Autodesk Fusion 360 part; units mm, degrees
sketch "Sketch1" plane through (0, 0, 0) normal (1, 0, 0) x (0, 1, 0)
  line L0 (0, 0) -> (35, 0)
  line L1 (35, 0) -> (35, -23)
  line L2 (35, -23) -> (40, -23)
  line L3 (0, 0) -> (0, 10)
  line L4 (15, 30.2) -> (15, 10)
  line L5 (15, 10) -> (40, 10)
  line L6 (40, 10) -> (40, -23)
  line L7 (0, 10) -> (0, 30)
  line L8 (0, 30) -> (0, 40)
  line L9 (0, 40) -> (15, 40)
  line L10 (15, 40) -> (15, 30.2)
  line L11 (15, 10) -> (15, 28.5) construction
  line L12 (15, 28.5) -> (35, 10)
  dimension "d1" = 35
  dimension "d2" = 23
  dimension "d3" = 5
  dimension "d4" = 10
  dimension "d8" = 20.2
  dimension "d9" = 20
  dimension "d10" = 10
  dimension "d19" = 18.5
extrude "Extrude1" add sketch "Sketch1" along normal blind 40 contours L0 L1 L2 L3 L4 L5 L6 L7 L8 L9 L10
sketch "Sketch2" plane through (0, 0, 0) normal (0, -1, 0) x (1, 0, 0)
  line L0 (0, 40) -> (0, 0)
  line L1 (0, 0) -> (40, 0)
  line L2 (40, 0) -> (40, 40)
  line L3 (40, 40) -> (0, 40)
  line L4 (29.815, 20) -> (24.9075, 28.5)
  line L5 (24.9075, 28.5) -> (15.0925, 28.5)
  line L6 (15.0925, 28.5) -> (10.185, 20)
  line L7 (10.185, 20) -> (15.0925, 11.5)
  line L8 (15.0925, 11.5) -> (24.9075, 11.5)
  line L9 (24.9075, 11.5) -> (29.815, 20)
  line L10 (0, 20) -> (40, 20) construction
  line L11 (20, 40) -> (20, 0) construction
  circle A0 centre (20, 20) radius 5.1
  line L12 (0, 0) -> (0, -11.5) construction
  line L13 (0, -11.5) -> (10, -11.5) construction
  line L14 (10, -11.5) -> (20, -11.5) construction
  circle A1 centre (20, -11.5) radius 2.1
  point P0 (20, 20)
  point P1 (20, 20)
  dimension "d13" = 8.5
  dimension "d14" = 10.2
  dimension "d25" = 11.5
  dimension "d26" = 10
  dimension "d27" = 4.2
extrude "Extrude2" cut sketch "Sketch2" against normal through all contours A0 | A1
extrude "Extrude3" cut sketch "Sketch2" along normal blind 7.5 from surface at -15 contours L4 L5 L6 L7 L8 L9
extrude "Extrude4" add sketch "Sketch1" along normal blind 4 contours L4 L5 L12
extrude "Extrude5" add sketch "Sketch1" against normal blind 4 from surface at 40 contours L4 L5 L12
sketch "Sketch3" plane through (0, 0, 10) normal (0, 0, 1) x (-1, 0, 0)
  line L0 (-36, -35) -> (-40, -35)
  line L1 (-40, -35) -> (-40, -40)
  line L2 (-40, -40) -> (0, -40)
  line L3 (0, -40) -> (0, -35)
  line L4 (0, -35) -> (-4, -35)
  line L5 (-4, -35) -> (-4, -15)
  line L6 (-4, -15) -> (-36, -15)
  line L7 (-36, -15) -> (-36, -35)
  line L8 (0, -40) -> (-10, -40) construction
  line L9 (-10, -40) -> (-10, -27.5) construction
  circle A0 centre (-10, -27.5) radius 1.6
  line L10 (-10, -27.5) -> (-30, -27.5) construction
  circle A1 centre (-30, -27.5) radius 1.6
  dimension "d28" = 10
  dimension "d29" = 12.5
  dimension "d30" = 3.2
  dimension "d31" = 20
  dimension "d32" = 3.2
extrude "Extrude6" cut sketch "Sketch3" along normal through all contours A0 | A1
equation "d8 = 30.200 mm - 10 mm"
equation "d13 = ( 17 / 2 ) * 1 mm"
equation "d19 = 28.50 mm - 10 mm"
equation "d25 = ( 23 / 2 ) * 1 mm"
equation "d29 = ( 25 / 2 ) * 1 mm"
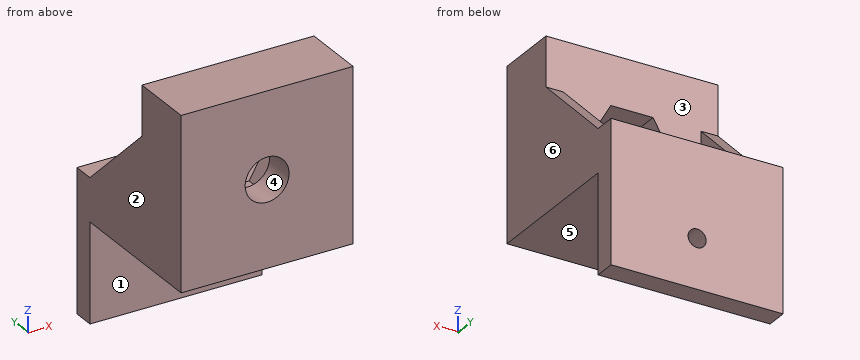
For this review, take the finished solid that the model builds, in its own axes (mm). Face numbers are marked on the shaded views. A direction names the side the tool comes from. Give positions to 0.01 mm unless a question says otherwise; leave off trailing zeros. Write each loop counter-clockwise with the first axis right and the second up, starting at its lowest first coordinate (ties: lowest second). Pieces come first, ordered by that corner, then holes. Notation, with made-up numbers: M 64,-31 L 119,-31 A24 cw 119,-21 Z; hole C 19.5,84 d6. An arc over 180 degrees is marked long. Answer as a JSON object with one key per item and string values. Group by question number.
Item 1: Consider section A-A on x = 20. Write out the cut boundary in (y, z).
Item 2: Consider section D-D on y = 27. Write out the cut boundary in (x, z), plus the area to 3 significant figures.
Item 3: Consider section B-B on y = 9.5. Write out the cut boundary in (x, z) (1 decimal), plus the area to 3 significant figures.
Item 4: Draft analysis for pull direction X (two halves, no side actions). For the marked faces 4, 5 and 6, state which applies: +X half, -X half, draft (parallel to the pull), parting line (faces both ways), or undercut.
Item 5: Consider section C-C on z = -11.5. Write out the cut boundary in (x, y).
Item 6: For probe 1 along Z at (x, y) = (20, 36.9); probe 2 along Z at (x, y) = (20, 2); probe 3 along X at (y, z) = (20.5, 17.5), list the stretches that pass through material, from the lowest coordinate up. Write a range as [from, to].
Item 7: For pin 1 Ø1 at (x, z) = (11.5, 16.5) entering from +Y; pin 2 Ø3 at (x, y) = (16.5, 20.5) entering from +Z; pin 3 Ø6 at (x, z) = (5.5, 14.5) entering from +Y, all flat-tipped, find the tip position at first contact; note any pin that passes through.
Item 8: Tool access review of the marked faces 1, 2 and 3: name each direction out of +Z, -Z, +X, -X, +Y, -Y from which nothing blocks a thin tool from reaching the whole face with its end or side.
Check result:
{
 "1": {"outline": "M 0,0 L 35,0 L 35,-9.4 L 40,-9.4 L 40,10 L 15,10 L 15,11.5 L 7.5,11.5 L 7.5,14.9 L 0,14.9 Z; M 0,25.1 L 7.5,25.1 L 7.5,28.5 L 15,28.5 L 15,40 L 0,40 Z; M 35,-23 L 40,-23 L 40,-13.6 L 35,-13.6 Z"},
 "2": {"outline": "M 0,0 L 40,0 L 40,17.4 L 36,17.4 L 36,10 L 4,10 L 4,17.4 L 0,17.4 Z", "area": "459 mm^2"},
 "3": {"outline": "M 0,0 L 40,0 L 40,40 L 0,40 Z; hole M 10.2,20 L 15.1,11.5 L 24.9,11.5 L 29.8,20 L 24.9,28.5 L 15.1,28.5 Z", "area": "1,350 mm^2"},
 "4": {"face 4": "undercut", "face 5": "draft", "face 6": "+X half"},
 "5": {"outline": "M 0,35 L 17.9,35 L 17.9,40 L 0,40 Z; M 22.1,35 L 40,35 L 40,40 L 22.1,40 Z"},
 "6": {"probe 1": "z = [-23, -13.6], [-9.4, 10]", "probe 2": "z = [0, 14.9], [25.1, 40]", "probe 3": "x = [0, 4], [36, 40]"},
 "7": {"pin 1": "stops at y = 15", "pin 2": "stops at z = 10", "pin 3": "stops at y = 32.94"},
 "8": {"face 1": "-Z, +X, -X, -Y", "face 2": "+Z, -Z, -X, +Y, -Y", "face 3": "+Z, +Y"}
}
